```python
from build123d import *

# Parameters (mm, degrees)
SKETCH1_W           = 58
SKETCH1_H           = 20
BOSS_EXTRUDE1_DEPTH = 10
SKETCH2_W           = 58
SKETCH2_H           = 10
BOSS_EXTRUDE3_DEPTH = 103
SKETCH4_W           = 58
SKETCH4_H           = 11
CUT_EXTRUDE2_DEPTH  = 103
SKETCH5_W           = 58
SKETCH5_H           = 31
BOSS_EXTRUDE4_DEPTH = 5
SKETCH6_W           = 58
SKETCH6_H           = 66.819677738
SKETCH6_W_2         = 58.198762754
SKETCH6_H_2         = 25.25
CUT_EXTRUDE3_DEPTH  = 5
FILLET2_START       = -39
FILLET2_DEPTH       = 58
FILLET2_2_DEPTH     = 58
FILLET3_R           = 2.5
SKETCH7_W           = 58.063983185
SKETCH7_H           = 11
CUT_EXTRUDE4_DEPTH  = 0.25
SKETCH9_R           = 3
SKETCH9_R_2         = 3.25
CUT_EXTRUDE5_DEPTH  = 139.455769111
FILLET4_R           = 5


with BuildPart() as part:
    # Sketch1 → Boss-Extrude1 (new body)
    with BuildSketch(Plane.XY):
        with Locations((-10, -19)):
            Rectangle(SKETCH1_W, SKETCH1_H)
    extrude(amount=BOSS_EXTRUDE1_DEPTH)

    # Sketch2 → Boss-Extrude3 (add)
    with BuildSketch(Plane.XZ.offset(29)):
        with Locations((-10, 5)):
            Rectangle(SKETCH2_W, SKETCH2_H)
    extrude(amount=BOSS_EXTRUDE3_DEPTH)

    # Sketch4 → Cut-Extrude2 (cut)
    with BuildSketch(Plane.XY.offset(10)):
        with Locations((-10, -91.25)):
            Rectangle(SKETCH4_W, SKETCH4_H)
    extrude(amount=-CUT_EXTRUDE2_DEPTH, mode=Mode.SUBTRACT)


with BuildPart() as cut_extrude2_piece_1:
    # of the separate pieces the step leaves, piece 1, a body of its own (cut_extrude2_pieces)
    add(part.part.solids().sort_by_distance((-39, -9, 0))[0])



with BuildPart() as cut_extrude2_piece_2:
    # of the separate pieces the step leaves, piece 2, a body of its own (cut_extrude2_pieces)
    add(part.part.solids().sort_by_distance((-39, -96.75, 10))[0])


with BuildPart() as cut_extrude2_piece_1_1:
    add(cut_extrude2_piece_1.part)

    add(cut_extrude2_piece_2.part)  # Boss-Extrude4 merges Cut-Extrude2 piece 2
    # Sketch5 → Boss-Extrude4 (add)
    with BuildSketch(Plane.XY.offset(10)):
        with Locations((-10, -91.25)):
            Rectangle(SKETCH5_W, SKETCH5_H)
    extrude(amount=BOSS_EXTRUDE4_DEPTH)

    # Sketch6 → Cut-Extrude3 (cut)
    with BuildSketch(Plane.XY.offset(10)):
        with Locations((-10, -42.340161131)):
            Rectangle(SKETCH6_W, SKETCH6_H)
        with Locations((-9.900618623, -119.375)):
            Rectangle(SKETCH6_W_2, SKETCH6_H_2)
    extrude(amount=-CUT_EXTRUDE3_DEPTH, mode=Mode.SUBTRACT)

    # Fillet2: read off the stored shape, not the designer's step
    # Fillet2 outline → Fillet2 (cut)
    with BuildSketch(Plane.YZ.offset(FILLET2_START)):
        with BuildLine():
            ThreePointArc((-106.75, 10), (-105.285533906, 13.535533906), (-101.75, 15))
            Line((-101.75, 15), (-106.75, 15))
            Line((-106.75, 15), (-106.75, 10))
        make_face()
        with BuildLine():
            ThreePointArc((-80.75, 15), (-77.214466094, 13.535533906), (-75.75, 10))
            Line((-75.75, 10), (-75.75, 15))
            Line((-75.75, 15), (-80.75, 15))
        make_face()
    extrude(amount=FILLET2_DEPTH, mode=Mode.SUBTRACT)

    # Fillet2 2 outline → Fillet2 2 (add)
    with BuildSketch(Plane.YZ.offset(FILLET2_START)):
        with BuildLine():
            Line((-75.75, 5), (-70.75, 5))
            ThreePointArc((-70.75, 5), (-74.285533906, 6.464466094), (-75.75, 10))
            Line((-75.75, 10), (-75.75, 5))
        make_face()
        with BuildLine():
            Line((-106.75, 5), (-106.75, 10))
            ThreePointArc((-106.75, 10), (-108.214466094, 6.464466094), (-111.75, 5))
            Line((-111.75, 5), (-106.75, 5))
        make_face()
    extrude(amount=FILLET2_2_DEPTH)

    # Fillet3
    fillet3_edges = [cut_extrude2_piece_1_1.edges().sort_by_distance(p)[0] for p in [
        (-10, -85.75, 0),
        (-10, -96.75, 0),
    ]]
    fillet(fillet3_edges, radius=FILLET3_R)

    # Sketch7 → Cut-Extrude4 (cut)
    with BuildSketch(Plane(origin=(0, 0, 10), x_dir=(-1, 0, 0), z_dir=(0, 0, -1))):
        with Locations((9.968008407, -91.25)):
            Rectangle(SKETCH7_W, SKETCH7_H)
    extrude(amount=-CUT_EXTRUDE4_DEPTH, mode=Mode.SUBTRACT)

    # Sketch9 → Cut-Extrude5 (cut, through all)
    with BuildSketch(Plane(origin=(0, 0, 0), x_dir=(-1, 0, 0), z_dir=(0, 0, -1))):
        with Locations((24.5, -17)):
            Circle(SKETCH9_R)
        with Locations((10, -17)):
            Circle(SKETCH9_R)
        with Locations((-4.5, -17)):
            Circle(SKETCH9_R)
        with Locations((31.5, -60.25)):
            Circle(SKETCH9_R_2)
        with Locations((31.5, -122.25)):
            Circle(SKETCH9_R_2)
    extrude(amount=-CUT_EXTRUDE5_DEPTH, mode=Mode.SUBTRACT)

    # Fillet4
    fillet4_edges = [cut_extrude2_piece_1_1.edges().sort_by_distance(p)[0] for p in [
        (-39, -9, 2.5),
        (19, -9, 2.5),
    ]]
    fillet(fillet4_edges, radius=FILLET4_R)


solid = cut_extrude2_piece_1_1.part
```
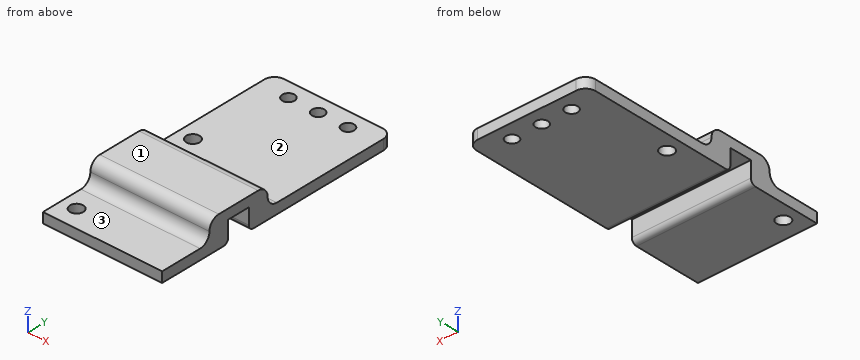
For this review, take the finished solid that the model builds, in its own axes (mm). Face numbers are marked on the shaded views. A direction names the side the tool comes from. Give positions to 0.01 mm unless a question says otherwise; leave off trailing zeros. Order: outer loops, then holes, each group sorted by start corner. A loop starts at its lowest first (then second) coordinate and runs counter-clockwise, first axis right, second up.
1) Insertion check: pin 1 (5.5 mm diameter, centred on x = 4.5, y = -17, fed in from -Z); pin 2 (3.5 mm diameter, centred on x = -2, y = -93, fed in from -Z); pin 3 (8.5 mm diameter, centred on x = -31.5, y = -122.25, fed in from +Z); pin 4 (12 mm diameter, centred on x = -6, y = -111.5, fed in from +Z). Each pin has a flat end and moves straight along its axis. Give the tip position at first contact, or say it passes through.
2) Take a section at A-A (y = -122.25). Give the boundary of the cut face in (x, z).
3) For the marked faces 1, 2 and 3, list the 3-axis set-ups (+Z, -Z, +X, -X, +Y, -Y) from which the entire face can be reached by the end or side of a thin tool; tool diameter is ignored.
4) Wall thickness on line 1 (Y direction, x = -6, z = 3.75); line 2 (Y direction, x = -26.5, z = 1); line 3 (Y direction, x = -29, z = 2.5): over which ranges is each line inside the solid? List them lowest first.
5) Take a section at B-B (x = -10). Give the boundary of the cut face in (y, z), then the cut area to 3 significant figures.
6) Take a section at C-C (y = -17). Give the boundary of the cut face in (x, z), then the cut area to 3 significant figures.
7) Take a section at D-D (z = 6.75). Give the boundary of the cut face in (x, y).
Derived:
1. pin 1: passes through
1. pin 2: stops at z = 10.25
1. pin 3: stops at z = 5
1. pin 4: stops at z = 13.31
2. outline: (-39, 0) - (-34.75, 0) - (-34.75, 5) - (-39, 5) - close; (-28.25, 0) - (19, 0) - (19, 5) - (-28.25, 5) - close
3. face 1: +Z, +X, -X, +Y, -Y
3. face 2: +Z, +X, -X, +Y
3. face 3: +Z, +X, -X, -Y
4. line 1: y = -132 to -96.75, -85.75 to -9
4. line 2: y = -132 to -97.25, -85.25 to -19.24, -14.76 to -9
4. line 3: y = -132 to -124.33, -120.17 to -96.75, -85.75 to -62.33, -58.17 to -9
5. outline: (-132, 0) - (-99.25, 0) arc R2.5 ccw to (-96.75, 2.5) - (-96.75, 10.25) - (-85.75, 10.25) - (-85.75, 2.5) arc R2.5 ccw to (-83.25, 0) - (-20, 0) - (-20, 5) - (-70.75, 5) arc R5 cw to (-75.75, 10) arc R5 ccw to (-80.75, 15) - (-101.75, 15) arc R5 ccw to (-106.75, 10) arc R5 cw to (-111.75, 5) - (-132, 5) - close; (-14, 0) - (-9, 0) - (-9, 5) - (-14, 5) - close
5. area: 780 mm2
6. outline: (-39, 0) - (-27.5, 0) - (-27.5, 5) - (-39, 5) - close; (-21.5, 0) - (-13, 0) - (-13, 5) - (-21.5, 5) - close; (-7, 0) - (1.5, 0) - (1.5, 5) - (-7, 5) - close; (7.5, 0) - (19, 0) - (19, 5) - (7.5, 5) - close
6. area: 200 mm2
7. outline: (-39, -107.95) - (19, -107.95) - (19, -96.75) - (-39, -96.75) - close; (-39, -85.75) - (19, -85.75) - (19, -74.55) - (-39, -74.55) - close
